from build123d import *

# Parameters (mm, degrees)
SKETCH1_R           = 1.6
BOSS_EXTRUDE1_DEPTH = 2
CUT_EXTRUDE1_DEPTH  = 2
SKETCH3_R           = 1.6
CUT_EXTRUDE2_DEPTH  = 2


with BuildPart() as part:
    # Sketch1 → Boss-Extrude1 (new body)
    with BuildSketch(Plane.XY):
        Polygon((21.467142273, 12.757289388), (98.986558646, 37.747522695), (108.606128903, 54.320788113), (91.526252569, 118.656423166), (69.674428961, 131.339810968), (5.135356345, 110.534101153), (-15.668691868, 74.691438373), align=None)
        with Locations((25.032859693, 16.533479235)):
            Circle(SKETCH1_R, mode=Mode.SUBTRACT)
        with Locations((-7.513458012, 70.813355701)):
            Circle(SKETCH1_R, mode=Mode.SUBTRACT)
        with Locations((68.212815702, 117.73514623)):
            Circle(SKETCH1_R, mode=Mode.SUBTRACT)
        Polygon((31.474266896, 21.347469407), (89.813558069, 36.835431526), (79.318927702, 76.366087142), (20.979636529, 60.878125023), align=None, mode=Mode.SUBTRACT)
    extrude(amount=BOSS_EXTRUDE1_DEPTH)

    # Sketch2 → Cut-Extrude1 (cut)
    with BuildSketch(Plane.XY.offset(2)):
        Polygon((68.505138354, 120.456079177), (89.039456874, 108.537406864), (105.056492564, 48.205227479), (108.606128903, 54.320788113), (91.526252569, 118.656423166), (69.674428961, 131.339810968), (5.135356345, 110.534101153), (-15.668691868, 74.691438373), (-13.318631122, 70.77207004), (3.322736479, 99.442976827), align=None)
    extrude(amount=-CUT_EXTRUDE1_DEPTH, mode=Mode.SUBTRACT)

    # Sketch3 → Cut-Extrude2 (cut)
    with BuildSketch(Plane.XY.offset(2)):
        with Locations((99.259718064, 45.190330298)):
            Circle(SKETCH3_R)
        with BuildLine():
            Line((6.456725485, 96.250579726), (64.230526779, 114.875342927))
            ThreePointArc((64.230526779, 114.875342927), (67.087527478, 113.411325508), (65.623510059, 110.554324808))
            Line((65.623510059, 110.554324808), (7.849708766, 91.929561608))
            ThreePointArc((7.849708766, 91.929561608), (4.992708066, 93.393579027), (6.456725485, 96.250579726))
        make_face()
        with BuildLine():
            Line((0.807577645, 86.517834494), (76.18470113, 110.817448579))
            ThreePointArc((76.18470113, 110.817448579), (79.041701829, 109.35343116), (77.57768441, 106.496430461))
            Line((77.57768441, 106.496430461), (2.200560925, 82.196816376))
            ThreePointArc((2.200560925, 82.196816376), (-0.656439775, 83.660833795), (0.807577645, 86.517834494))
        make_face()
        with BuildLine():
            Line((-3.419178071, 77.243631299), (83.571572672, 105.287175206))
            ThreePointArc((83.571572672, 105.287175206), (86.428573372, 103.823157787), (84.964555952, 100.966157087))
            Line((84.964555952, 100.966157087), (-2.02619479, 72.92261318))
            ThreePointArc((-2.02619479, 72.92261318), (-4.88319549, 74.3866306), (-3.419178071, 77.243631299))
        make_face()
        with BuildLine():
            Line((-3.448967162, 69.322420425), (85.506365232, 97.999294098))
            ThreePointArc((85.506365232, 97.999294098), (88.363365932, 96.535276679), (86.899348513, 93.678275979))
            Line((86.899348513, 93.678275979), (-2.055983882, 65.001402307))
            ThreePointArc((-2.055983882, 65.001402307), (-4.912984581, 66.465419726), (-3.448967162, 69.322420425))
        make_face()
        with BuildLine():
            Line((-0.651479152, 62.312649778), (87.441157792, 90.71141299))
            ThreePointArc((87.441157792, 90.71141299), (90.298158492, 89.247395571), (88.834141073, 86.390394871))
            Line((88.834141073, 86.390394871), (0.741504129, 57.991631659))
            ThreePointArc((0.741504129, 57.991631659), (-2.115496571, 59.455649078), (-0.651479152, 62.312649778))
        make_face()
        with BuildLine():
            Line((83.038019838, 81.380348772), (89.375950353, 83.423531882))
            ThreePointArc((89.375950353, 83.423531882), (92.232951052, 81.959514463), (90.768933633, 79.102513764))
            Line((90.768933633, 79.102513764), (84.431003119, 77.059330653))
            ThreePointArc((84.431003119, 77.059330653), (81.574002419, 78.523348073), (83.038019838, 81.380348772))
        make_face()
        with BuildLine():
            Line((3.323909307, 55.682603442), (15.979695788, 59.762498153))
            ThreePointArc((15.979695788, 59.762498153), (18.836696487, 58.298480734), (17.372679068, 55.441480034))
            Line((17.372679068, 55.441480034), (4.716892588, 51.361585323))
            ThreePointArc((4.716892588, 51.361585323), (1.859891888, 52.825602742), (3.323909307, 55.682603442))
        make_face()
        with BuildLine():
            Line((7.299297766, 49.052557106), (17.914488348, 52.474617045))
            ThreePointArc((17.914488348, 52.474617045), (20.771489047, 51.010599626), (19.307471628, 48.153598926))
            Line((19.307471628, 48.153598926), (8.692281046, 44.731538987))
            ThreePointArc((8.692281046, 44.731538987), (5.835280347, 46.195556407), (7.299297766, 49.052557106))
        make_face()
        with BuildLine():
            Line((11.274686225, 42.42251077), (19.849280908, 45.186735937))
            ThreePointArc((19.849280908, 45.186735937), (22.706281607, 43.722718518), (21.242264188, 40.865717818))
            Line((21.242264188, 40.865717818), (12.667669505, 38.101492652))
            ThreePointArc((12.667669505, 38.101492652), (9.810668805, 39.565510071), (11.274686225, 42.42251077))
        make_face()
        with BuildLine():
            Line((15.250074683, 35.792464434), (21.784073468, 37.898854829))
            ThreePointArc((21.784073468, 37.898854829), (24.641074168, 36.43483741), (23.177056748, 33.577836711))
            Line((23.177056748, 33.577836711), (16.643057964, 31.471446316))
            ThreePointArc((16.643057964, 31.471446316), (13.786057264, 32.935463735), (15.250074683, 35.792464434))
        make_face()
        with BuildLine():
            Line((19.225463142, 29.162418098), (23.718866028, 30.610973721))
            ThreePointArc((23.718866028, 30.610973721), (26.575866728, 29.146956302), (25.111849309, 26.289955603))
            Line((25.111849309, 26.289955603), (20.618446422, 24.84139998))
            ThreePointArc((20.618446422, 24.84139998), (17.761445723, 26.305417399), (19.225463142, 29.162418098))
        make_face()
        with BuildLine():
            Line((84.972812398, 74.092467664), (91.310742913, 76.135650774))
            ThreePointArc((91.310742913, 76.135650774), (94.167743612, 74.671633355), (92.703726193, 71.814632656))
            Line((92.703726193, 71.814632656), (86.365795679, 69.771449546))
            ThreePointArc((86.365795679, 69.771449546), (83.508794979, 71.235466965), (84.972812398, 74.092467664))
        make_face()
        with BuildLine():
            Line((86.907604959, 66.804586556), (93.245535473, 68.847769666))
            ThreePointArc((93.245535473, 68.847769666), (96.102536172, 67.383752247), (94.638518753, 64.526751548))
            Line((94.638518753, 64.526751548), (88.300588239, 62.483568438))
            ThreePointArc((88.300588239, 62.483568438), (85.44358754, 63.947585857), (86.907604959, 66.804586556))
        make_face()
        with BuildLine():
            Line((88.842397519, 59.516705448), (95.180328033, 61.559888559))
            ThreePointArc((95.180328033, 61.559888559), (98.037328733, 60.095871139), (96.573311314, 57.23887044))
            Line((96.573311314, 57.23887044), (90.235380799, 55.19568733))
            ThreePointArc((90.235380799, 55.19568733), (87.3783801, 56.659704749), (88.842397519, 59.516705448))
        make_face()
        with BuildLine():
            Line((90.777190079, 52.228824341), (97.115120593, 54.272007451))
            ThreePointArc((97.115120593, 54.272007451), (99.972121293, 52.807990032), (98.508103874, 49.950989332))
            Line((98.508103874, 49.950989332), (92.170173359, 47.907806222))
            ThreePointArc((92.170173359, 47.907806222), (89.31317266, 49.371823641), (90.777190079, 52.228824341))
        make_face()
    extrude(amount=-CUT_EXTRUDE2_DEPTH, mode=Mode.SUBTRACT)


solid = part.part
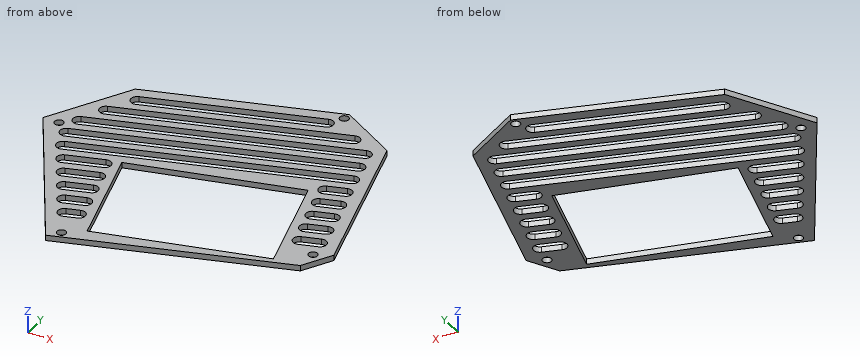
Can you work these out from the model? Positions are in its coordinate system, mm. Give positions to 0.01 mm unless a question says otherwise; leave off trailing zeros. Loops run counter-clockwise (first coordinate to the right, second up) from the corner with the lowest first, then second, coordinate; pieces in that order, holes last. Notation, with made-up numbers: (29.5, -33) - (71.5, -33) arc R18 cw to (71.5, -21) - close; hole circle Ø1 at (18.5, -27.75). An arc over 180 degrees is marked (long way). Answer as a JSON object with one key per item and string values.
Q1. If I drill on L1, parallel to X at y = 41, z = 0.55; L2, parallel to Y at x = 75, z = 0.3; L3, parallel to Y at x = 0, z = 0.8, over which ranges is the centre line in solid material (lowest first)?
Geometry says:
{"L1": "4.53 to 9.82, 21.57 to 26.26, 88.71 to 100.87", "L2": "30.01 to 32.9, 75.22 to 81.93, 86.7 to 89.84, 94.61 to 97.75, 102.52 to 105.67, 110.44 to 116.69", "L3": "48.56 to 57.88, 62.52 to 65.66, 70.43 to 73.58, 78.35 to 82.66, 86.06 to 93.72"}
Q2. Imagine slicing it at B-B on z = 0.9. Give the number of separate pieces and of enclosed holes in the cut face, plus the area to 3 significant figures.
Geometry says:
{"separate pieces": "1", "enclosed holes": "20", "area": "3,520 mm²"}
Q3. Will this pin go through, and if not, where does the flat tip stop? P1, Ø2.5, axis at x = -7.51, y = 70.81, coming from the -Z side.
Geometry says:
{"P1": "through"}
Q4. Imagine slicing it at A-A on x = 42.5. Write out the boundary of the cut face in (y, z), plus the area to 3 significant figures.
Geometry says:
{"outline": "(19.54, 0) - (24.27, 0) - (24.27, 2) - (19.54, 2) - close; (66.59, 0) - (71.45, 0) - (71.45, 2) - (66.59, 2) - close; (76.22, 0) - (79.37, 0) - (79.37, 2) - (76.22, 2) - close; (84.14, 0) - (87.28, 0) - (87.28, 2) - (84.14, 2) - close; (92.05, 0) - (95.19, 0) - (95.19, 2) - (92.05, 2) - close; (99.96, 0) - (103.1, 0) - (103.1, 2) - (99.96, 2) - close; (107.87, 0) - (112.07, 0) - (112.07, 2) - (107.87, 2) - close", "area": "52.7 mm²"}
